The listing builds one solid part. Answer for the finished solid, in the listing's coordinates (mm). A direction names the side the tool comes from. Give positions to 0.01 mm unless a question says otherwise; leave off trailing zeros. Order: outer loops, then holes, each group sorted by start corner. A loop starts at its lowest first (then second) coordinate and runs counter-clockwise, first axis right, second up. Notation, with made-up numbers: (60.25, -15) - (80.25, -15) arc R8 cw to (80.25, -8) - close; hole circle Ø1 at (53, 59). An arc over 180 degrees is marked (long way). Write each question's results on one line, items separated by ' | '. Start each with the question number.
1. Which of the six approach directions +Z, -Z, +X, -X, +Y, -Y give full straight-line access (tool end or side, diameter ignored) to faces 1 (the face through (507, 239.3, -98.9)), 2 (the face through (507, 249.3, 7.8)), 3 (the face through (945.92, 109.08, 4.93)), 4 (the face through (507, -239.3, 108.9))?
2. Determine the mould class of faces 5 (the face through (54.61, 229.13, 4.93)), 6 (the face through (507, -249.3, 2.2)), 7 (the face through (1000, 2, 5)), 8 (the face through (54.063, -194.146, 4.93)) for opening direction Y: released by +Y, released by -Y, zero draft, split by the parting line, or undercut.
3. Flat-ended cylindrical pins translate along their axes: pin 1 (1.5 mm diameter, centred on x = 537, z = 150.5, fed in from -Y) (3 decimals); pin 2 (8 mm diameter, centred on x = 709.5, y = 197.5, fed in from -Z); pin 3 (1.5 mm diameter, centred on x = 316, z = -108.5, fed in from +Y) (3 decimals). Find the tip coordinate at first contact, or state that the pin passes through.
4. Section B-B (y = -12) is taken. State how many separate pieces and enclosed holes the cut face has, and give its area (3 significant figures).
5. Find the intervals of material crossed by L1, parallel to Y at x = 145, z = -50; L2, parallel to Y at x = 824.5, z = 1.5; L3, parallel to Y at x = 77, z = 66.5, in increasing order.
6. Section A-A (z = -67) is taken. Give the vertices of the cut face in (x, y), and give its area (3 significant figures).
from build123d import *

# Parameters (mm, degrees)
CUT_EXTRUDE2_DEPTH = 1076.127215203


with BuildPart() as part:
    # Sketch1 → Loft4 section 0
    with BuildSketch(Plane(origin=(0, 0, 0), x_dir=(0, 0, -1), z_dir=(1, 0, 0))):
        Polygon((-205, 300), (195, 300), (195, 290), (0, 290), (0, -290), (195, -290), (195, -300), (-205, -300), (-205, -290), (-10, -290), (-10, 290), (-205, 290), align=None)
    # Sketch4 → Loft4 section 1
    with BuildSketch(Plane(origin=(1000, 0, -1000), x_dir=(0, 0, 1), z_dir=(-1, 0, 0))):
        Polygon((805, 200), (1205, 200), (1205, 190), (1010, 190), (1010, -190), (1205, -190), (1205, -200), (805, -200), (805, -190), (1000, -190), (1000, 190), (805, 190), align=None)
    loft()

    # 3DSketch1 → Cut-Extrude2 (cut, through all)
    with BuildSketch(Plane(origin=(955, -149.275559705, 0), x_dir=(-0.9193091385176674, 0.39353615823441734, 0), z_dir=(0, 0, 1))):
        with BuildLine():
            Line((23.771900268, 13.114838789), (651.375957176, 359.360866092))
            ThreePointArc((651.375957176, 359.360866092), (676.975392867, 353.930952286), (675.287892891, 327.816446442))
            Line((675.287892891, 327.816446442), (127.715549412, -228.2676011))
            ThreePointArc((127.715549412, -228.2676011), (109.754280938, -233.887743911), (95.078586754, -222.105674031))
            Line((95.078586754, -222.105674031), (10.684359853, -24.958900083))
            ThreePointArc((10.684359853, -24.958900083), (9.89296563, -3.400627082), (23.771900268, 13.114838789))
        make_face()
        with BuildLine():
            Line((825.502793093, 383.974217556), (976.828190217, 30.474754914))
            ThreePointArc((976.828190217, 30.474754914), (976.508407209, 6.141893153), (958.252169109, -9.948482636))
            Line((958.252169109, -9.948482636), (220.359519027, -242.09716271))
            ThreePointArc((220.359519027, -242.09716271), (197.283607657, -233.434785068), (200.139914384, -208.95262863))
            Line((200.139914384, -208.95262863), (792.899174378, 390.169926603))
            ThreePointArc((792.899174378, 390.169926603), (810.850417384, 395.751870528), (825.502793093, 383.974217556))
        make_face()
    extrude(amount=CUT_EXTRUDE2_DEPTH, mode=Mode.SUBTRACT)


solid = part.part
Reported:
1) face 1: -Z, -X | face 2: +Z, -Z, +X, +Y | face 3: +Z, -Z | face 4: +Z, -X
2) face 5: undercut | face 6: released by -Y | face 7: zero draft | face 8: undercut
3) pin 1: y = -246.375 | pin 2: z = 0 | pin 3: y = 268.475
4) separate pieces: 3 | enclosed holes: 0 | area: 1,930 mm²
5) L1: -285.5 to -275.5, 275.5 to 285.5 | L2: -217.55 to -162.33, 68.69 to 109.89, 162.33 to 217.55 | L3: -292.3 to -282.3, 282.3 to 292.3
6) outline: (0, -300) - (1000, -200) - (1000, -190) - (0, -290) - close; (0, 290) - (1000, 190) - (1000, 200) - (0, 300) - close | area: 20,000 mm²
